Could you check a few things on this model? Use its own coordinates, in mm. Face numbers are marked on the shaded views. Give positions to 0.01 mm unless a question says otherwise; leave off trailing zeros. Write each loop counter-clockwise with the first axis right and the second up, starting at its lowest first coordinate (ties: lowest second). Pieces come first, ordered by that corner, then holes. Notation, with made-up numbers: (67, 10) - (124, 10) arc R15 ccw to (124, 25) - close; hole circle Ø1 at (-33, 30). An arc over 180 degrees is marked (long way). Write item = value, one per line.
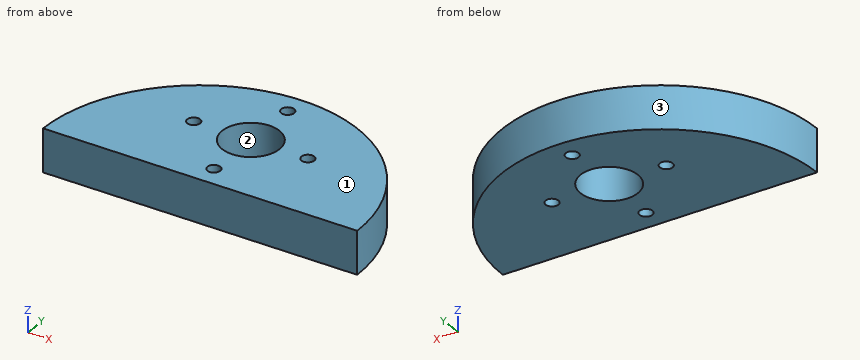
from build123d import *

# Parameters (mm, degrees)
BOSS_EXTRU_2_DEPTH      = 6
ESQUISSE4_R             = 4
ESQUISSE4_R_2           = 0.9
ENL_V_MAT_EXTRU_1_DEPTH = 6


with BuildPart() as part:
    # Esquisse2 → Boss.-Extru.2 (new body)
    with BuildSketch(Plane.XY):
        with BuildLine():
            Line((-22, 0), (22, 0))
            ThreePointArc((22, 0), (0, 22), (-22, 0))
        make_face()
    extrude(amount=BOSS_EXTRU_2_DEPTH)

    # Esquisse4 → Enlèv. mat.-Extru.1 (cut)
    with BuildSketch(Plane(origin=(0, 0, 0), x_dir=(-1, 0, 0), z_dir=(0, 0, -1))):
        with Locations((0, 11)):
            Circle(ESQUISSE4_R)
        with Locations((0, 19)):
            Circle(ESQUISSE4_R_2)
        with Locations((0, 3)):
            Circle(ESQUISSE4_R_2)
        with Locations((-8, 11)):
            Circle(ESQUISSE4_R_2)
        with Locations(Location((8, 11, 0), (0, 0, 180))):
            Circle(ESQUISSE4_R_2)
    extrude(amount=-ENL_V_MAT_EXTRU_1_DEPTH, mode=Mode.SUBTRACT)


solid = part.part
1. If we section it at A-A, the plane x = 0: Please give me the cut outline in (y, z), and give its area (3 significant figures).
Filled sheet:
outline = (0, 0) - (2.1, 0) - (2.1, 6) - (0, 6) - close; (3.9, 0) - (7, 0) - (7, 6) - (3.9, 6) - close; (15, 0) - (18.1, 0) - (18.1, 6) - (15, 6) - close; (19.9, 0) - (22, 0) - (22, 6) - (19.9, 6) - close
area = 62.4 mm2
2. If we section it at B-B, the plane z = 0.95: Please give me the cut outline in (x, y), and give its area (3 significant figures).
Filled sheet:
outline = (-22, 0) - (22, 0) arc R22 ccw to start; hole circle Ø1.8 at (-8, 11); hole circle Ø8 at (0, 11); hole circle Ø1.8 at (0, 3); hole circle Ø1.8 at (0, 19); hole circle Ø1.8 at (8, 11)
area = 700 mm2
3. I need wall thicknesses on line 1 (Y direction, x = 0, z = 3.2); line 2 (X direction, y = 7.75, z = 4.45); line 3 (X direction, y = 11.5, z = 1.9) (3 decimals). Which ranges of each line are inside material? Lowest first, please.
Filled sheet:
line_1 = 0 to 2.1, 3.9 to 7, 15 to 18.1, 19.9 to 22
line_2 = -20.59 to -2.33, 2.33 to 20.59
line_3 = -18.755 to -8.748, -7.252 to -3.969, 3.969 to 7.252, 8.748 to 18.755
4. For pin 1 (1.1 mm diameter, centred on x = 0, y = 19, fed in from -Z); pin 2 (1 mm diameter, centred on y = 16, z = 4, fed in from -X); pin 3 (3 mm diameter, centred on y = 12, z = 5, fed in from +X), each with a flat end and sliding along its axis, tell me the tip position at first contact or that it passes through.
Filled sheet:
pin_1 = through
pin_2 = -15.61
pin_3 = 19.33
5. If we section it at D-D, the plane x = -8: Please give me the cut outline in (y, z).
Filled sheet:
outline = (0, 0) - (10.1, 0) - (10.1, 6) - (0, 6) - close; (11.9, 0) - (20.49, 0) - (20.49, 6) - (11.9, 6) - close
6. Thinking about a two-plate mould opening in X: for the marked faces 1, 2 and 3, which applies, pulls with the +X half, pulls with the -X half, needs draft (parallel to the pull), parting line crosses it, or undercut?
Filled sheet:
face_1 = needs draft
face_2 = undercut
face_3 = parting line crosses it
7. If we section it at C-C, the plane y = 3: Please give me the cut outline in (x, z).
Filled sheet:
outline = (-21.79, 0) - (-0.9, 0) - (-0.9, 6) - (-21.79, 6) - close; (0.9, 0) - (21.79, 0) - (21.79, 6) - (0.9, 6) - close
